Model file for the job. Use its own axes, mm. Round coordinates to 2 decimals unless told otherwise and drop trailing zeros. Loops run counter-clockwise (first coordinate to the right, second up) from the corner with the lowest first, then second, coordinate; pieces in that order, holes last. Notation, with made-up numbers: M 79,-7 L 136,-7 A18 ccw 136,13 Z; hole C 15,39.5 d7. An arc over 180 degrees is marked long. Answer in a Markdown table with one row per item.
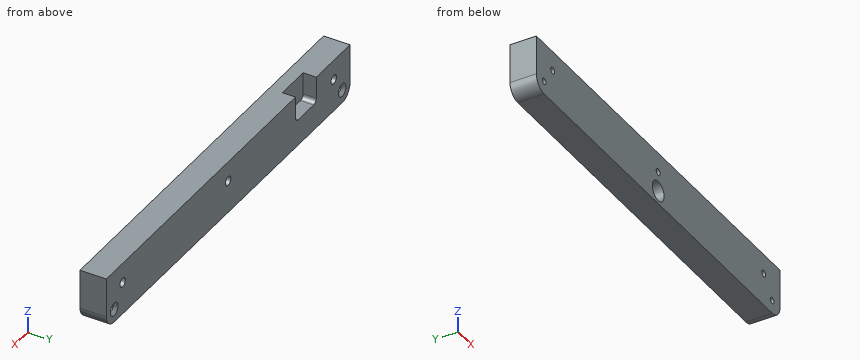
from build123d import *

# Parameters (mm, degrees)
SKETCH1_W           = 298.45
SKETCH1_H           = 38.1
BOSS_EXTRUDE1_DEPTH = 19.05
FILLET1_R           = 9.525
SKETCH2_R           = 3.302
CUT_EXTRUDE1_DEPTH  = 14.2875
SKETCH4_R           = 1.4224
CUT_EXTRUDE2_DEPTH  = 302.47456775
SKETCH5_R           = 2.413
CUT_EXTRUDE3_DEPTH  = 2.921
SKETCH6_R           = 2.1844
CUT_EXTRUDE4_DEPTH  = 302.47456775
CHAMFER1_SIZE       = 2.54
CHAMFER1_SIZE2      = 2.207988314
CUT_EXTRUDE5_START  = -5.08
SKETCH7_R           = 7.239
CUT_EXTRUDE5_DEPTH  = 297.39456775
CUT_EXTRUDE6_START  = -9.525
SKETCH8_W           = 25.4
SKETCH8_H           = 19.05
CUT_EXTRUDE6_DEPTH  = 9.525
FILLET2_R           = 3.175


with BuildPart() as part:
    # Sketch1 → Boss-Extrude1 (new body)
    with BuildSketch(Plane(origin=(0, 0, 0), x_dir=(1, 0, 0), z_dir=(0, 1, 0))):
        with Locations((149.225, 19.05)):
            Rectangle(SKETCH1_W, SKETCH1_H)
    extrude(amount=BOSS_EXTRUDE1_DEPTH)

    # Fillet1
    fillet1_edges = [part.edges().sort_by_distance(p)[0] for p in [
        (0, 9.525, -38.1),
        (298.45, 9.525, -38.1),
    ]]
    fillet(fillet1_edges, radius=FILLET1_R)

    # Sketch2 → Cut-Extrude1 (cut)
    with BuildSketch(Plane(origin=(0, 19.05, 0), x_dir=(1, 0, 0), z_dir=(0, 1, 0))):
        with Locations(Location((19.939, 14.351, 0), (0, 0, 270))):
            Circle(SKETCH2_R)
        with Locations(Location((149.225, 14.351, 0), (0, 0, 270))):
            Circle(SKETCH2_R)
        with Locations(Location((278.511, 14.351, 0), (0, 0, 270))):
            Circle(SKETCH2_R)
    extrude(amount=-CUT_EXTRUDE1_DEPTH, mode=Mode.SUBTRACT)

    # Sketch4 → Cut-Extrude2 (cut, through all)
    with BuildSketch(Plane.XZ):
        with Locations(Location((19.939, -14.351, 0), (0, 0, 270))):
            Circle(SKETCH4_R)
        with Locations(Location((149.225, -14.351, 0), (0, 0, 270))):
            Circle(SKETCH4_R)
        with Locations(Location((278.511, -14.351, 0), (0, 0, 270))):
            Circle(SKETCH4_R)
    extrude(amount=-CUT_EXTRUDE2_DEPTH, mode=Mode.SUBTRACT)

    # Sketch5 → Cut-Extrude3 (cut)
    with BuildSketch(Plane.XZ):
        with Locations(Location((19.939, -14.351, 0), (0, 0, 270))):
            Circle(SKETCH5_R)
        with Locations(Location((149.225, -14.351, 0), (0, 0, 270))):
            Circle(SKETCH5_R)
        with Locations(Location((278.511, -14.351, 0), (0, 0, 270))):
            Circle(SKETCH5_R)
    extrude(amount=-CUT_EXTRUDE3_DEPTH, mode=Mode.SUBTRACT)

    # Sketch6 → Cut-Extrude4 (cut, through all)
    with BuildSketch(Plane(origin=(0, 19.05, 0), x_dir=(1, 0, 0), z_dir=(0, 1, 0))):
        with BuildLine():
            ThreePointArc((286.7406, 28.575), (288.925, 26.3906), (291.1094, 28.575))
            Line((291.1094, 28.575), (286.7406, 28.575))
        make_face()
        with BuildLine():
            Line((286.7406, 28.575), (291.1094, 28.575))
            ThreePointArc((291.1094, 28.575), (288.925, 30.7594), (286.7406, 28.575))
        make_face()
        with Locations(Location((9.525, 28.575, 0), (0, 0, 270))):
            Circle(SKETCH6_R)
    extrude(amount=-CUT_EXTRUDE4_DEPTH, mode=Mode.SUBTRACT)

    # Chamfer1
    chamfer1_edges = [part.edges().sort_by_distance(p)[0] for p in [
        (291.1094, 19.05, -28.575),
        (9.525, 19.05, -30.7594),
    ]]
    chamfer1_side = [part.faces().sort_by_distance(p)[0] for p in [
        (149.225, 19.05, -19.008778326),
    ]]
    chamfer(chamfer1_edges, length=CHAMFER1_SIZE, length2=CHAMFER1_SIZE2, reference=chamfer1_side[0])

    # Sketch7 → Cut-Extrude5 (cut, through all)
    with BuildSketch(Plane(origin=(0, 19.05, 0), x_dir=(1, 0, 0), z_dir=(0, 1, 0)).offset(CUT_EXTRUDE5_START)):
        with Locations(Location((149.225, 28.575, 0), (0, 0, 270))):
            Circle(SKETCH7_R)
    extrude(amount=-CUT_EXTRUDE5_DEPTH, mode=Mode.SUBTRACT)

    # Sketch8 → Cut-Extrude6 (cut)
    with BuildSketch(Plane.XZ.offset(CUT_EXTRUDE6_START)):
        with Locations((53.975, -9.525)):
            Rectangle(SKETCH8_W, SKETCH8_H)
    extrude(amount=-CUT_EXTRUDE6_DEPTH, mode=Mode.SUBTRACT)

    # Fillet2
    fillet2_edges = [part.edges().sort_by_distance(p)[0] for p in [
        (41.275, 14.2875, -19.05),
        (66.675, 14.2875, -19.05),
    ]]
    fillet(fillet2_edges, radius=FILLET2_R)


solid = part.part
1. Pin check, flat tips, straight feed: pin 1 (7 mm diameter, centred on x = 148.5, z = -27.5, fed in from -Y); pin 2 (4 mm diameter, centred on x = 278.511, z = -14.351, fed in from +Y); pin 3 (1.5 mm diameter, centred on y = 8, z = -34, fed in from -X); pin 4 (7.5 mm diameter, centred on x = 279.5, z = -13, fed in from +Y). Stop position of each tip, or through.
Verdict:
| item | result |
|---|---|
| pin 1 | stops at y = 13.97 |
| pin 2 | stops at y = 4.76 |
| pin 3 | stops at x = 1.23 |
| pin 4 | stops at y = 19.05 |
2. Saw through at A-A (z = -6.5). Write the cut outline in (x, y) (3 decimals).
Verdict:
| item | result |
|---|---|
| outline | M 0,0 L 298.45,0 L 298.45,19.05 L 66.675,19.05 L 66.675,9.525 L 41.275,9.525 L 41.275,19.05 L 0,19.05 Z |
3. Wall check: probe 1 along X at (y, z) = (14.25, -16); probe 2 along X at (y, z) = (2, -28); probe 3 along X at (y, z) = (12.75, -12) (3 decimals). Give the ranges that are in metal, low to high.
Verdict:
| item | result |
|---|---|
| probe 1 | x = 0 to 17.08, 22.8 to 41.28, 66.67 to 146.36, 152.09 to 275.65, 281.37 to 298.45 |
| probe 2 | x = 0 to 7.42, 11.63 to 142.01, 156.44 to 286.82, 291.03 to 298.45 |
| probe 3 | x = 0 to 17.62, 22.258 to 41.275, 66.675 to 146.906, 151.544 to 276.192, 280.83 to 298.45 |
4. Saw through at B-B (x = 55). Write the cut outline in (y, z) (3 decimals), and give its area (3 significant figures).
Verdict:
| item | result |
|---|---|
| outline | M 0,-38.1 L 19.05,-38.1 L 19.05,-19.05 L 9.525,-19.05 L 9.525,0 L 0,0 Z |
| area | 544 mm² |
